Autodesk Inventor part; units mm, degrees
ref_plane "YZ Plane" through (0, 0, 0) normal (1, 0, 0) x (0, 1, 0)
ref_plane "XZ Plane" through (0, 0, 0) normal (0, 1, 0) x (-1, 0, 0)
ref_plane "XY Plane" through (0, 0, 0) normal (0, 0, 1) x (1, 0, 0)
sketch "Sketch1" plane through (0, 0, 0) normal (0, 0, 1) x (1, 0, 0)
  line L0 (0, 0) -> (-3.45, 0)
  line L1 (-3.45, 0) -> (-3.45, -20)
  line L2 (-3.45, -20) -> (0, -20)
  line L3 (0, -20) -> (0, 0)
  line L4 (-1.725, -20) -> (-5.425, -20)
  line L5 (-5.425, -20) -> (1.925, -20)
  line L6 (1.925, -20) -> (1.925, -25)
  line L7 (1.925, -25) -> (-5.425, -25)
  line L8 (-5.425, -25) -> (-5.425, -20)
  dimension "d0" = 20
  dimension "d1" = 3.45
  dimension "d2" = 3.7
  dimension "d3" = 7.35
  dimension "d4" = 5
extrude "Extrusion1" add sketch "Sketch1" along normal blind 3.5
sketch "Sketch4" plane through (0, 0, 0) normal (0, 0, -1) x (-1, 0, 0)
  line L0 (0, -20) -> (0, 0)
  line L1 (-1.925, -20) -> (0, -20)
  line L2 (-1.925, -25) -> (-1.925, -20)
  line L3 (5.425, -25) -> (-1.925, -25)
  line L4 (5.425, -20) -> (5.425, -25)
  line L5 (3.45, -20) -> (5.425, -20)
  line L6 (3.45, 0) -> (3.45, -20)
  line L7 (0, 0) -> (3.45, 0)
  line L8 (3.45, 0) -> (5.475, 0)
  line L9 (0, 0) -> (-2.025, 0)
  line L10 (5.475, 0) -> (-2.025, 0)
  line L11 (-2.025, 0) -> (-2.025, 4)
  line L12 (-2.025, 4) -> (5.475, 4)
  line L13 (5.475, 4) -> (5.475, 0)
  circle A0 centre (1.725, 4) radius 3.75
  circle A1 centre (1.725, 4) radius 1.55
  dimension "d22" = 2.025
  dimension "d23" = 2.025
  dimension "d24" = 7.5
  dimension "d25" = 4
  dimension "d26" = 3.1
extrude "Extrusion4" add sketch "Sketch4" against normal up to surface (3.5 mm away) contours L9 L11 A0 L13 L8 L7 | A0 L12 A1 | L12 A1 A0
sketch "Sketch5" plane through (0, 0, 0) normal (0, 0, -1) x (-1, 0, 0)
  circle A0 centre (1.725, 4) radius 1.55
  line L0 (0, -20) -> (0, 0)
  line L1 (-1.925, -20) -> (0, -20)
  line L2 (-1.925, -25) -> (-1.925, -20)
  line L3 (5.425, -25) -> (-1.925, -25)
  line L4 (5.425, -20) -> (5.425, -25)
  line L5 (3.45, -20) -> (5.425, -20)
  line L6 (3.45, 0) -> (3.45, -20)
  line L7 (3.45, 0) -> (5.475, 0)
  line L8 (5.475, 0) -> (5.475, 4)
  arc A1 (5.475, 4) -> (-2.025, 4) centre (1.725, 4) ccw
  line L9 (-2.025, 4) -> (-2.025, 0)
  line L10 (-2.025, 0) -> (0, 0)
  line L11 (3.45, -10) -> (0, -10)
  line L12 (2.45, -10) -> (2.45, -20)
  line L13 (1, -10) -> (1, -20)
  line L14 (3.45, -20) -> (2.45, -20)
  line L15 (1, -20) -> (0, -20)
  dimension "d29" = 1
  dimension "d30" = 1
extrude "Extrusion5" cut sketch "Sketch5" against normal up to surface (3.5 mm away) contours L0 L11 L13 L15 | L0 L10 L9 A1 L8 L7 L6 L11 | L11 L6 L14 L12
sketch "Sketch6" plane through (0, 0, 3.5) normal (0, 0, 1) x (1, 0, 0)
  line L0 (1.925, -20) -> (-1, -20)
  line L1 (-1, -20) -> (-1, -10)
  line L2 (-1, -10) -> (-2.45, -10)
  line L3 (-2.45, -10) -> (-2.45, -20)
  line L4 (-2.45, -20) -> (-5.425, -20)
  line L5 (-5.425, -20) -> (-5.425, -25)
  line L6 (-5.425, -25) -> (1.925, -25)
  line L7 (1.925, -25) -> (1.925, -20)
  line L8 (-1, -20) -> (-2.45, -20)
  point P0 (0, 0)
extrude "Extrusion6" cut sketch "Sketch6" against normal blind 1.75 contours L8 L3 L2 L1
sketch "Sketch7" plane through (-5.425, -20, 3.5) normal (0, 1, 0) x (1, 0, 0)
  line L0 (4.425, 3.5) -> (7.35, 3.5)
  line L1 (4.425, 3.5) -> (4.425, 1.75)
  line L2 (4.425, 1.75) -> (2.975, 1.75)
  line L3 (2.975, 3.5) -> (2.975, 1.75)
  line L4 (0, 3.5) -> (2.975, 3.5)
  line L5 (0, 3.5) -> (0, 0)
  line L6 (7.35, 0) -> (0, 0)
  line L7 (7.35, 3.5) -> (7.35, 0)
  line L8 (0.5, 0.5) -> (0.5, 3)
  line L9 (0.5, 3) -> (2.475, 3)
  line L10 (2.475, 3) -> (2.475, 1.25)
  line L11 (2.475, 1.25) -> (4.925, 1.25)
  line L12 (4.925, 1.25) -> (4.925, 3)
  line L13 (4.925, 3) -> (6.85, 3)
  line L14 (6.85, 3) -> (6.85, 0.5)
  line L15 (6.85, 0.5) -> (0.5, 0.5)
  line L16 (2.475, 3) -> (4.925, 3)
  line L17 (2.975, 3.5) -> (4.425, 3.5)
  point P0 (5.425, 3.5)
  dimension "d35" = 0.5
extrude "Extrusion7" cut sketch "Sketch7" along normal blind 10 and the other way blind 2 contours L0 L7 L6 L5 L4 L3 L16 L9 L8 L15 L14 L13 L1 | L1 L16 L3 L17
sketch "Sketch8" plane through (-5.425, -22, 3.5) normal (0, 1, 0) x (1, 0, 0)
  line L0 (0, 3.5) -> (7.35, 3.5)
  line L1 (0, 0) -> (0, 3.5)
  line L2 (7.35, 0) -> (0, 0)
  line L3 (7.35, 3.5) -> (7.35, 0)
  line L4 (6.85, 3) -> (0.5, 3)
  line L5 (6.85, 0.5) -> (6.85, 3)
  line L6 (0.5, 0.5) -> (6.85, 0.5)
  line L7 (0.5, 3) -> (0.5, 0.5)
  point P0 (5.425, 3.5)
extrude "Extrusion8" add sketch "Sketch8" along normal up to surface (2 mm away)
sketch "Sketch9" plane through (-5.425, -20, 0) normal (0, 1, 0) x (1, 0, 0)
  line L0 (0, 0) -> (7.35, 0)
  line L1 (0, -3.5) -> (0, 0)
  line L2 (7.35, -3.5) -> (0, -3.5)
  line L3 (7.35, 0) -> (7.35, -3.5)
  line L4 (4.425, -0.5) -> (2.975, -0.5)
  line L5 (4.425, -0.5) -> (4.425, -1.75)
  line L6 (4.425, -1.75) -> (2.975, -1.75)
  line L7 (2.975, -0.5) -> (2.975, -1.75)
  line L8 (4.425, -0.5) -> (4.425, 0)
  line L9 (2.975, -0.5) -> (2.975, 0)
  point P0 (5.425, 0)
extrude "Extrusion9" add sketch "Sketch9" along normal blind 10 contours L0 L8 L4 L9
sketch "Sketch10" plane through (0, 0, 1.75) normal (0, 0, 1) x (1, 0, 0)
  line L0 (-1, -20) -> (-2.45, -20)
  line L1 (-1, -10) -> (-1, -20)
  line L2 (-2.45, -10) -> (-1, -10)
  line L3 (-2.45, -20) -> (-2.45, -10)
  point P0 (0, 0)
extrude "Extrusion10" add sketch "Sketch10" along normal up to surface (1.75 mm away)
sketch "Sketch11" plane through (-2.45, -10, 0) normal (0, 1, 0) x (1, 0, 0)
  line L0 (0, 0) -> (0, -3.5)
  line L1 (0, -3.5) -> (1.45, -3.5)
  line L2 (1.45, 0) -> (1.45, -3.5)
  line L3 (1.45, 0) -> (0, 0)
  point P0 (2.45, 0)
extrude "Extrusion11" add sketch "Sketch11" along normal blind 10
sketch "Sketch12" plane through (0, 0, 3.5) normal (0, 0, 1) x (1, 0, 0)
  line L0 (-5.425, -20) -> (-5.425, -25)
  line L1 (-5.425, -25) -> (1.925, -25)
  line L2 (1.925, -25) -> (1.925, -20)
  line L3 (1.925, -20) -> (-1, -20)
  line L4 (-1, -20) -> (-1, 0)
  line L5 (-2.45, 0) -> (-1, 0)
  line L6 (-2.45, -20) -> (-2.45, 0)
  line L7 (-2.45, -20) -> (-5.425, -20)
  line L8 (-1.75, -25) -> (-5.425, -25)
  line L9 (-5.425, -25) -> (-5.325, -25)
  line L10 (-5.325, -25) -> (-5.325, -20)
  line L11 (-1.75, -25) -> (1.925, -25)
  line L12 (1.925, -25) -> (1.825, -25)
  line L13 (1.825, -25) -> (1.825, -20)
  point P0 (0, 0)
  dimension "d48" = 0.1
  dimension "d49" = 0.1
extrude "Extrusion12" cut sketch "Sketch12" against normal up to surface (3.5 mm away) contours L7 L10 L1 L0 | L13 L3 L2 L1
sketch "Sketch17" plane through (0, 0, 3.5) normal (0, 0, 1) x (1, 0, 0)
  line L0 (1.825, -25) -> (1.825, -20)
  line L1 (1.825, -20) -> (-1, -20)
  line L2 (-1, -20) -> (-1, 0)
  line L3 (-2.45, 0) -> (-1, 0)
  line L4 (-2.45, -20) -> (-2.45, 0)
  line L5 (-2.45, -20) -> (-5.325, -20)
  line L6 (-5.325, -20) -> (-5.325, -25)
  line L7 (-5.325, -25) -> (1.825, -25)
  line L8 (-1, -20) -> (-2.45, -20)
  point P0 (0, 0)
extrude "Extrusion17" cut sketch "Sketch17" against normal blind 1 contours L8 L4 L3 L2
sketch "Sketch18" plane through (0, 0, 3.5) normal (0, 0, 1) x (1, 0, 0)
  line L0 (1.825, -20) -> (-5.325, -20)
  line L1 (-5.325, -20) -> (-5.325, -25)
  line L2 (-5.325, -25) -> (1.825, -25)
  line L3 (1.825, -25) -> (1.825, -20)
  line L4 (1.825, -25) -> (1.675, -25)
  line L5 (1.675, -25) -> (1.675, -20)
  line L6 (-5.325, -25) -> (-5.175, -25)
  line L7 (-5.175, -25) -> (-5.175, -20)
  point P0 (0, 0)
  dimension "d65" = 0.15
  dimension "d66" = 0.15
extrude "Extrusion18" cut sketch "Sketch18" against normal up to surface (3.5 mm away) contours L3 L2 L5 L0 | L7 L2 L1 L0
sketch "Sketch19" plane through (0, 0, 2.5) normal (0, 0, 1) x (1, 0, 0)
  line L0 (-2.45, 0) -> (-1, 0)
  line L1 (-2.45, -20) -> (-2.45, 0)
  line L2 (-1, -20) -> (-2.45, -20)
  line L3 (-1, 0) -> (-1, -20)
  line L4 (-1.725, 0) -> (-2.45, 0)
  line L5 (-2.45, 0) -> (-2.3, 0)
  line L6 (-2.3, 0) -> (-2.3, -20)
  line L7 (-1, -20) -> (-1.15, -20)
  line L8 (-1.15, -20) -> (-1.15, 0)
  point P0 (0, 0)
  dimension "d69" = 0.15
  dimension "d70" = 0.15
extrude "Extrusion19" cut sketch "Sketch19" against normal up to surface (2.5 mm away) contours L0 L6 L2 L1 | L0 L3 L2 L8
equation "\"d23\" = d22"
equation "\"d30\" = d29"
equation "\"d49\" = d48"
equation "\"d69\" = d70"
properties part number "Piston"
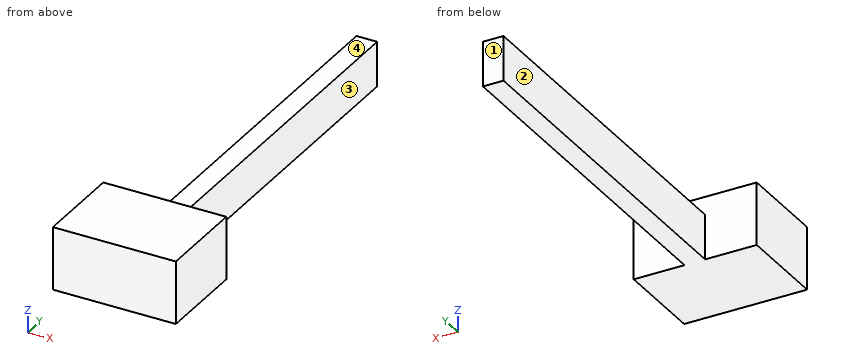
Source: CAD feature listing. Evaluate the final solid. Frame: model axes, mm. Face numbers are marked on the shaded views. A direction names the side the tool comes from. Give positions to 0.01 mm unless a question says otherwise; leave off trailing zeros. Write each loop counter-clockwise with the first axis right and the second up, starting at its lowest first coordinate (ties: lowest second). Pieces come first, ordered by that corner, then holes. Notation, with made-up numbers: (-3.75, 71.25) - (31.25, 71.25) arc R16 cw to (31.25, 92.25) - close; hole circle Ø9 at (43, -25). An arc over 180 degrees is marked (long way). Write item = value, one per line. Start each with the question number.
Q1. Material intervals for probe 1 along Y at (x, z) = (-2.75, 0.3); probe 2 along X at (y, z) = (-16.5, 1.5); probe 3 along Z at (x, y) = (-2, -17.25), sorted ascending.
Q2. Reachability of the marked faces 1, 2, 3 and 4 from +Z, -Z, +X, -X, +Y, -Y: full face, straight path, thin tool, end or side. Return the list, or none.
Q3. Cut plane D-D, the plane x = -3.75. Return loops of the section in (y, z), then the cut area to 3 significant figures.
Q4. Cut plane B-B, the plane x = -1.5. Return loops of the section in (y, z).
Q5. Cut plane A-A, the plane z = 1.8. Return loops of the section in (x, y) (3 decimals).
Q6. Cut plane C-C, the plane y = -15.25. Return loops of the section in (x, z).
Q7. Pin query (flat end, axial travel): pin 1 Ø2 at (x, y) = (-2.5, -18.5) entering from +Z; pin 2 Ø0.8 at (y, z) = (-13.5, 1.5) entering from +X; pin 3 Ø0.8 at (y, z) = (-7, 1.5) entering from -X. Return the tip coordinate at first contact, or that it passes through.
Computed values:
q1.probe_1 = -25 to -20
q1.probe_2 = -2.3 to -1.15
q1.probe_3 = 0 to 2.5
q2.face_1 = +Z, -Z, +X, -X, +Y
q2.face_2 = +Z, -Z, -X, +Y
q2.face_3 = +Z, -Z, +X, +Y
q2.face_4 = +Z, +X, -X, +Y
q3.outline = (-25, 0) - (-20, 0) - (-20, 3.5) - (-25, 3.5) - close
q3.area = 17.5 mm²
q4.outline = (-25, 0) - (0, 0) - (0, 2.5) - (-20, 2.5) - (-20, 3.5) - (-25, 3.5) - close
q5.outline = (-5.175, -25) - (1.675, -25) - (1.675, -20) - (-1.15, -20) - (-1.15, 0) - (-2.3, 0) - (-2.3, -20) - (-5.175, -20) - close
q6.outline = (-2.3, 0) - (-1.15, 0) - (-1.15, 2.5) - (-2.3, 2.5) - close
q7.pin_1 = 2.5
q7.pin_2 = -1.15
q7.pin_3 = -2.3
